Answer from the drawing. Dimensions are ordinates in mm from the lowest x, y and z of the part. Round coordinates to 2 decimals unless told otherwise and drop trailing zeros. Write each loop counter-clockwise with the first axis right and the second up, starting at its lowest first coordinate (ties: lowest second). Pieces come first, ordered by that corner, then holes. Notation, with made-up numbers: (60.5, 21) - (75.5, 21) arc R15 cw to (75.5, 26) - close; hole circle Ø2 at (-14.75, 56). An arc over 180 degrees is marked (long way). Answer as CSV lines item,"result". Start each with the question number.
1) Consider line 1 along Z through (x, y) = (23, 1.15); line 2 along Z through (x, y) = (23, 30.5); line 3 along Y through (x, z) = (15.5, 25). Determine where each line is inside the solid, lowest interval first.
2) Find section B-B on z = 20. Determine the outline of the cut face in (x, y), then the cut area to 3 significant figures.
3) Find section A-A on x = 23. Determine the outline of the cut face in (y, z).
4) Each of these flat-tipped pins is pushed along its axis until it touches: pin 1 (15.5 mm diameter, centred on x = 23, z = 20, fed in from +Y); pin 2 (15.5 mm diameter, centred on x = 22.5, z = 21, fed in from -Y). Where does it stop, or does it pass through?
5) Find section D-D on z = 13. Determine the outline of the cut face in (x, y).
6) For a pull along Z with two mould halves and no side action, classify the marked faces 1, 2 and 3 as +Z half, -Z half, draft (parallel to the pull), parting line (faces both ways), or undercut.
7) Find section C-C on y = 27.5. Determine the outline of the cut face in (x, z), then the cut area to 3 significant figures.
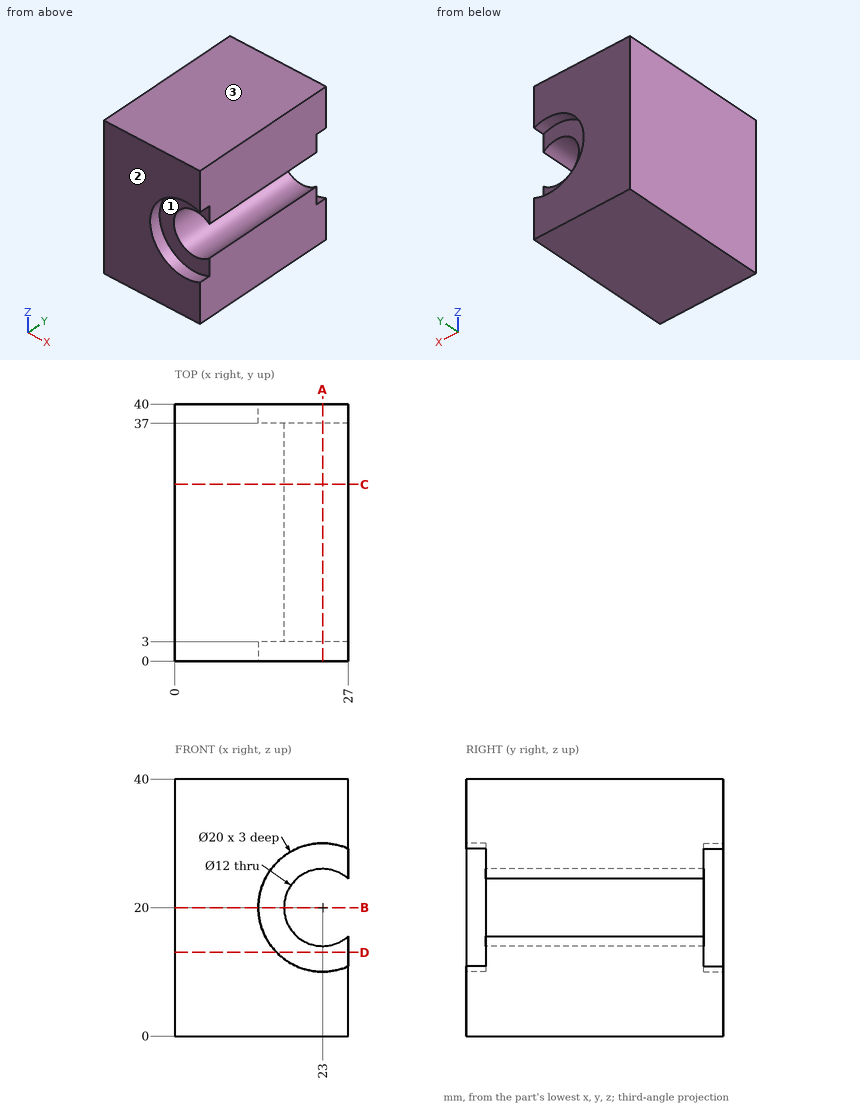
Check values:
1,line 1,"z = 0 to 10, 30 to 40"
1,line 2,"z = 0 to 14, 26 to 40"
1,line 3,"y = 3 to 37"
2,outline,"(0, 0) - (13, 0) - (13, 3) - (17, 3) - (17, 37) - (13, 37) - (13, 40) - (0, 40) - close"
2,area,"656 mm^2"
3,outline,"(0, 0) - (40, 0) - (40, 10) - (37, 10) - (37, 14) - (3, 14) - (3, 10) - (0, 10) - close; (0, 30) - (3, 30) - (3, 26) - (37, 26) - (37, 30) - (40, 30) - (40, 40) - (0, 40) - close"
4,pin 1,"stops at y = 37"
4,pin 2,"stops at y = 3"
5,outline,"(0, 0) - (15.86, 0) - (15.86, 3) - (27, 3) - (27, 37) - (15.86, 37) - (15.86, 40) - (0, 40) - close"
6,face 1,"undercut"
6,face 2,"draft"
6,face 3,"+Z half"
7,outline,"(0, 0) - (27, 0) - (27, 15.53) arc R6 cw (long way) to (27, 24.47) - (27, 40) - (0, 40) - close"
7,area,"979 mm^2"
